```python
from build123d import *

# Parameters (mm, degrees)
ESQUISSE1_W             = 12
ESQUISSE1_H             = 188
BOSS_EXTRU_1_DEPTH      = 4
ESQUISSE2_R             = 2
BOSS_EXTRU_2_DEPTH      = 30
ESQUISSE3_W             = 12
ESQUISSE3_H             = 188
BOSS_EXTRU_3_DEPTH      = 4
ENL_V_MAT_EXTRU_1_DEPTH = 74
ENL_V_MAT_EXTRU_2_DEPTH = 74
ENL_V_START             = -74
ESQUISSE6_R             = 2
ENL_V_MAT_EXTRU_3_DEPTH = 74
ESQUISSE8_W             = 4
ESQUISSE8_H             = 36
BOSS_EXTRU_4_DEPTH      = 30
ESQUISSE7_R             = 2
ENL_V_MAT_EXTRU_6_DEPTH = 193.177001746


with BuildPart() as part:
    # Esquisse1 → Boss.-Extru.1 (new body)
    with BuildSketch(Plane.XY):
        with Locations((6, 94)):
            Rectangle(ESQUISSE1_W, ESQUISSE1_H)
    extrude(amount=BOSS_EXTRU_1_DEPTH)

    # Esquisse2 → Boss.-Extru.2 (add)
    with BuildSketch(Plane.XY.offset(4)):
        with Locations(Location((6, 182, 0), (0, 0, 180))):
            Circle(ESQUISSE2_R)
        with Locations(Location((6, 6, 0), (0, 0, 180))):
            Circle(ESQUISSE2_R)
    extrude(amount=BOSS_EXTRU_2_DEPTH)

    # Esquisse3 → Boss.-Extru.3 (add)
    with BuildSketch(Plane.XY.offset(34)):
        with Locations((6, 94)):
            Rectangle(ESQUISSE3_W, ESQUISSE3_H)
    extrude(amount=BOSS_EXTRU_3_DEPTH)

    # Esquisse4 → Enlèv. mat.-Extru.1 (cut)
    with BuildSketch(Plane.XY.offset(38)):
        with BuildLine():
            Line((0, 182), (0, 193.947131368))
            Line((0, 193.947131368), (12, 193.947131368))
            Line((12, 193.947131368), (12, 182))
            ThreePointArc((12, 182), (6, 188), (0, 182))
        make_face()
    extrude(amount=-ENL_V_MAT_EXTRU_1_DEPTH, mode=Mode.SUBTRACT)

    # Esquisse5 → Enlèv. mat.-Extru.2 (cut)
    with BuildSketch(Plane.XY.offset(38)):
        with BuildLine():
            Line((12, 6), (12, -5.88895182))
            Line((12, -5.88895182), (0, -5.88895182))
            Line((0, -5.88895182), (0, 6))
            ThreePointArc((0, 6), (6, 0), (12, 6))
        make_face()
    extrude(amount=-ENL_V_MAT_EXTRU_2_DEPTH, mode=Mode.SUBTRACT)

    # Esquisse6 → Enlèv. mat.-Extru.3 (cut)
    with BuildSketch(Plane.XY.offset(38).offset(ENL_V_START)):
        with Locations((6, 6)):
            Circle(ESQUISSE6_R)
    extrude(amount=ENL_V_MAT_EXTRU_3_DEPTH, mode=Mode.SUBTRACT)

    # Esquisse8 → Boss.-Extru.4 (add)
    with BuildSketch(Plane.XY.offset(4)):
        with Locations((6, 94)):
            Rectangle(ESQUISSE8_W, ESQUISSE8_H)
    extrude(amount=BOSS_EXTRU_4_DEPTH)

    # Esquisse7 → Enlèv. mat.-Extru.6 (cut, through all)
    with BuildSketch(Plane.XY.offset(38)):
        with Locations((6, 182)):
            Circle(ESQUISSE7_R)
    extrude(amount=-ENL_V_MAT_EXTRU_6_DEPTH, mode=Mode.SUBTRACT)


solid = part.part
```
Could you check a few things on this model? Use its own coordinates, in mm. A direction names the side the tool comes from. Round coordinates to 2 decimals unless told otherwise and drop trailing zeros. Order: outer loops, then holes, each group sorted by start corner. A loop starts at its lowest first (then second) coordinate and runs counter-clockwise, first axis right, second up. Notation, with made-up numbers: M 40,-2 L 85,-2 A27 cw 85,19 Z; hole C 75.25,68 d11. An arc over 180 degrees is marked long. One line per question, with ' | ' between items. Start each with the question number.
(1) For P1, Ø10, axis at y = 113, z = 25, coming from the +X side; P2, Ø5, axis at x = 7.5, z = 22.5, coming from the +Y side; P3, Ø6, axis at x = 7.5, z = 20.5, coming from the -Y side, each with a flat end and sliding along its axis, tell me the tip position at first contact or that it passes through.
(2) For faces 5 (the face through (8, 94, 19)), 6 (the face through (6, 112, 19)), 7 (the face through (6, 76, 19)), 8 (the face through (12, 93, 2)), which set-ups out of +Z, -Z, +X, -X, +Y, -Y let a thin tool reach every point of the face, with its end or its side?
(3) Suppose I cut it at B-B on x = 6. List the corners of the cut face in (y, z) for me.
(4) Suppose I cut it at C-C on z = 17.5. List the corners of the cut face in (x, y) for me.
(5) Thinking about a two-plate mould opening in Z: for faces 1 (the face through (4, 94, 19)), 2 (the face through (6, 0, 2)), 3 (the face through (6, 95, 38)), 4 (the face through (6, 95, 0)), which applies, +Z half, -Z half, draft (parallel to the pull), parting line (faces both ways), or undercut?
(6) Suppose I cut it at A-A on y = 165. List the corners of the cut face in (x, z) for me, then the cut area to 3 significant figures.
(7) Please list where these lines run through material, in increasing order: line 1 along Y through (x, z) = (6, 1.9); line 2 along Z through (x, y) = (4.5, 61.5); line 3 along X through (y, z) = (182, 35.85).
Geometry results:
1) P1: x = 8 | P2: y = 112 | P3: y = 76
2) face 5: +X, +Y, -Y | face 6: +X, -X, +Y | face 7: +X, -X, -Y | face 8: +Z, -Z, +X, +Y, -Y
3) outline: M 0,0 L 4,0 L 4,4 L 0,4 Z; M 0,34 L 4,34 L 4,38 L 0,38 Z; M 8,0 L 180,0 L 180,4 L 112,4 L 112,34 L 180,34 L 180,38 L 8,38 L 8,34 L 76,34 L 76,4 L 8,4 Z; M 184,0 L 188,0 L 188,4 L 184,4 Z; M 184,34 L 188,34 L 188,38 L 184,38 Z
4) outline: M 4,76 L 8,76 L 8,112 L 4,112 Z
5) face 1: undercut | face 2: draft | face 3: +Z half | face 4: -Z half
6) outline: M 0,0 L 12,0 L 12,4 L 0,4 Z; M 0,34 L 12,34 L 12,38 L 0,38 Z | area: 96.0 mm²
7) line 1: 0 to 4, 8 to 180, 184 to 188 | line 2: 0 to 4, 34 to 38 | line 3: 0 to 4, 8 to 12
